from build123d import *

# Parameters (mm, degrees)
BOSS_EXTRUDE1_DEPTH = 304.8
SKETCH4_W           = 12.7
SKETCH4_H           = 6.223
CUT_EXTRUDE1_DEPTH  = 306.114409233
LPATTERN1_COUNT     = 24
LPATTERN1_PITCH     = 25.4
BOSS_EXTRUDE2_DEPTH = 609.6
SKETCH6_W           = 12.7
SKETCH6_H           = 6.223
CUT_EXTRUDE2_DEPTH  = 306.114409233
LPATTERN2_COUNT     = 24
LPATTERN2_PITCH     = 25.4
SKETCH7_R           = 1.5875
BOSS_EXTRUDE3_DEPTH = 609.6
CHAMFER1_SIZE       = 0.3175
CUT_EXTRUDE3_START  = -88.9
SKETCH8_W           = 11.762471384
SKETCH8_H           = 30.066276354
CUT_EXTRUDE3_DEPTH  = 521.857265411
FILLET1_R           = 3.175
SKETCH9_R           = 2.032
CUT_EXTRUDE4_DEPTH  = 306.162001268


with BuildPart() as part:
    # Sketch3 → Boss-Extrude1 (new, symmetric)
    with BuildSketch(Plane(origin=(0, 0, 0), x_dir=(0, 0, -1), z_dir=(1, 0, 0))):
        with BuildLine():
            Line((1.5875, 0), (1.5875, -2.676056053))
            Line((1.5875, -2.676056053), (1.5875, -13.49375))
            Line((1.5875, -13.49375), (3.1115, -13.49375))
            Line((3.1115, -13.49375), (3.1115, 0))
            ThreePointArc((3.1115, 0), (-2.624212484, 1.671807731), (1.314976721, -2.819976679))
            Line((1.314976721, -2.819976679), (0.670906491, -1.438763612))
            ThreePointArc((0.670906491, -1.438763612), (-1.33888392, 0.852963128), (1.5875, 0))
        make_face()
    extrude(amount=BOSS_EXTRUDE1_DEPTH, both=True)

    # Sketch4 → Cut-Extrude1 (cut, symmetric)
    with BuildSketch(Plane.XY):
        with Locations((298.45, 0)):
            Rectangle(SKETCH4_W, SKETCH4_H)
    cut_extrude1 = extrude(amount=CUT_EXTRUDE1_DEPTH, both=True, mode=Mode.SUBTRACT)

    # LPattern1: Cut-Extrude1 ×24
    with Locations(*[(-i * LPATTERN1_PITCH, 0, 0) for i in range(1, LPATTERN1_COUNT)]):
        add(cut_extrude1, mode=Mode.SUBTRACT)


with BuildPart() as body_2:
    # Sketch5 → Boss-Extrude2 (new body)
    with BuildSketch(Plane(origin=(304.8, 0, 0), x_dir=(0, 0, -1), z_dir=(1, 0, 0))):
        with BuildLine():
            Line((1.5875, 13.49375), (1.5875, 2.676056053))
            Line((1.5875, 2.676056053), (1.5875, 0))
            ThreePointArc((1.5875, 0), (-1.33888392, -0.852963128), (0.670906491, 1.438763612))
            Line((0.670906491, 1.438763612), (1.314976721, 2.819976679))
            ThreePointArc((1.314976721, 2.819976679), (-2.624212484, -1.671807731), (3.1115, 0))
            Line((3.1115, 0), (3.1115, 13.49375))
            Line((3.1115, 13.49375), (1.5875, 13.49375))
        make_face()
    extrude(amount=-BOSS_EXTRUDE2_DEPTH)

    # Sketch6 → Cut-Extrude2 (cut, symmetric)
    with BuildSketch(Plane.XY):
        with Locations((285.75, 0)):
            Rectangle(SKETCH6_W, SKETCH6_H)
    cut_extrude2 = extrude(amount=CUT_EXTRUDE2_DEPTH, both=True, mode=Mode.SUBTRACT)

    # LPattern2: Cut-Extrude2 ×24
    with Locations(*[(-i * LPATTERN2_PITCH, 0, 0) for i in range(1, LPATTERN2_COUNT)]):
        add(cut_extrude2, mode=Mode.SUBTRACT)


with BuildPart() as body_3:
    # Sketch7 → Boss-Extrude3 (new body)
    with BuildSketch(Plane(origin=(304.8, 0, 0), x_dir=(0, 0, -1), z_dir=(1, 0, 0))):
        Circle(SKETCH7_R)
    extrude(amount=-BOSS_EXTRUDE3_DEPTH)

    # Chamfer1
    chamfer1_edges = [body_3.edges().sort_by_distance(p)[0] for p in [
        (304.8, 0, 1.5875),
        (-304.8, 0, 1.5875),
    ]]
    chamfer(chamfer1_edges, length=CHAMFER1_SIZE)


with BuildPart() as cut_extrude3_tool:
    # Sketch8 → Cut-Extrude3 (new, through all)
    with BuildSketch(Plane.ZY.offset(304.8).offset(CUT_EXTRUDE3_START)):
        Rectangle(SKETCH8_W, SKETCH8_H)
    extrude(amount=-CUT_EXTRUDE3_DEPTH)


with BuildPart() as part_1:
    add(part.part)

    # Cut-Extrude3: cut by cut_extrude3_tool
    add(cut_extrude3_tool.part, mode=Mode.SUBTRACT)

    # Fillet1
    fillet1_edges = [part_1.edges().sort_by_distance(p)[0] for p in [
        (-215.9, -13.49375, -2.3495),
        (-304.8, -13.49375, -2.3495),
    ]]
    fillet(fillet1_edges, radius=FILLET1_R)

    # Sketch9 → Cut-Extrude4 (cut, through all)
    with BuildSketch(Plane(origin=(0, 0, -3.1115), x_dir=(-1, 0, 0), z_dir=(0, 0, -1))):
        with Locations(Location((222.25, -8.73125, 0), (0, 0, 90))):
            Circle(SKETCH9_R)
        with Locations(Location((298.45, -8.73125, 0), (0, 0, 90))):
            Circle(SKETCH9_R)
    extrude(amount=-CUT_EXTRUDE4_DEPTH, mode=Mode.SUBTRACT)


with BuildPart() as body_2_1:
    add(body_2.part)

    # Cut-Extrude3: cut by cut_extrude3_tool
    add(cut_extrude3_tool.part, mode=Mode.SUBTRACT)


with BuildPart() as body_3_1:
    add(body_3.part)

    # Cut-Extrude3: cut by cut_extrude3_tool
    add(cut_extrude3_tool.part, mode=Mode.SUBTRACT)


solid = part_1.part
Model file for the job. Use its own axes, mm. A direction names the side the tool comes from. Coordinates: 2 decimals unless noted, no trailing zeros. Write each loop counter-clockwise with the first axis right and the second up, starting at its lowest first coordinate (ties: lowest second). Pieces come first, ordered by that corner, then holes. Notation, with made-up numbers: (3.25, -5.5) -> (61.25, -5.5) arc R16 cw to (61.25, -1.5) -> close; hole circle Ø5 at (43, 35). An arc over 180 degrees is marked (long way). One line per item, written item: value. Start each with the question number.
1) Flat gauge pins, fed straight in: pin 1 Ø1.2 at (x, z) = (-236, -2) entering from +Y; pin 2 Ø6.5 at (x, y) = (-261.5, -9.5) entering from +Z; pin 3 Ø2 at (y, z) = (-11.5, -1.5) entering from +X. Where does each tip first touch, or does it go through?
2) Which spindle directions (+Z, -Z, +X, -X, +Y, -Y) get a long thin tool onto all of the face, cutting with end or side? Do faces 1 (the face through (-272.96, -2.14, -1)), 2 (the face through (-300.434, -9.172, -2.36)), 3 (the face through (-292.1, 1.3, -1.3)). Say none if no direction does.
3) Slice it at D-D on x = -232.5. Write the cut outline in (y, z).
4) Pull direction Z, two halves, no side cores. Call faces 4 (the face through (-260, -7, -3.112)), 5 (the face through (-215.9, -2.2, -0.6)), 6 (the face through (-247.56, 0.8, 1.37)), 7 (the face through (-222.16, 0.8, 1.37)): +Z half, -Z half, draft (parallel to the pull), parting line (faces both ways), or undercut.
5) Slice it at C-C on y = -4.25. Write the cut outline in (x, z), then the cut area to 3 significant figures.
6) Slice it at B-B on x = -247.5. Write the cut outline in (y, z) (1 decimal).
7) Slice it at A-A on x = -222.25. Write the cut outline in (y, z) (1 decimal).
8) Probe probe 1 along X at (y, z) = (1.5, 2); probe 2 along Z at (x, y) = (-248.5, 0); probe 3 along Z at (x, y) = (-274.5, -5.75). List the from-to ranges inside material, lowest first.
Answers follow:
1. pin 1: y = -3.11
1. pin 2: z = -1.59
1. pin 3: x = -215.91
2. face 1: +X, -X
2. face 2: +Z, -Z
2. face 3: +Z, -Z, +Y
3. outline: (-13.49, -3.11) -> (-3.11, -3.11) -> (-3.11, -1.59) -> (-13.49, -1.59) -> close
4. face 4: -Z half
4. face 5: draft
4. face 6: undercut
4. face 7: undercut
5. outline: (-304.8, -3.11) -> (-215.9, -3.11) -> (-215.9, -1.59) -> (-304.8, -1.59) -> close
5. area: 135 mm2
6. outline: (-13.5, -3.1) -> (0, -3.1) arc R3.1 ccw (long way) to (-2.8, -1.3) -> (-1.4, -0.7) arc R1.6 cw (long way) to (0, -1.6) -> (-13.5, -1.6) -> close
7. outline: (-13.5, -3.1) -> (-10.8, -3.1) -> (-10.8, -1.6) -> (-13.5, -1.6) -> close; (-6.7, -3.1) -> (0, -3.1) arc R3.1 ccw (long way) to (-2.8, -1.3) -> (-1.4, -0.7) arc R1.6 cw (long way) to (0, -1.6) -> (-6.7, -1.6) -> close
8. probe 1: -304.8 to -292.1, -279.4 to -266.7, -254 to -241.3, -228.6 to -215.9
8. probe 2: -3.11 to -1.59, 1.59 to 3.11
8. probe 3: -3.11 to -1.59
